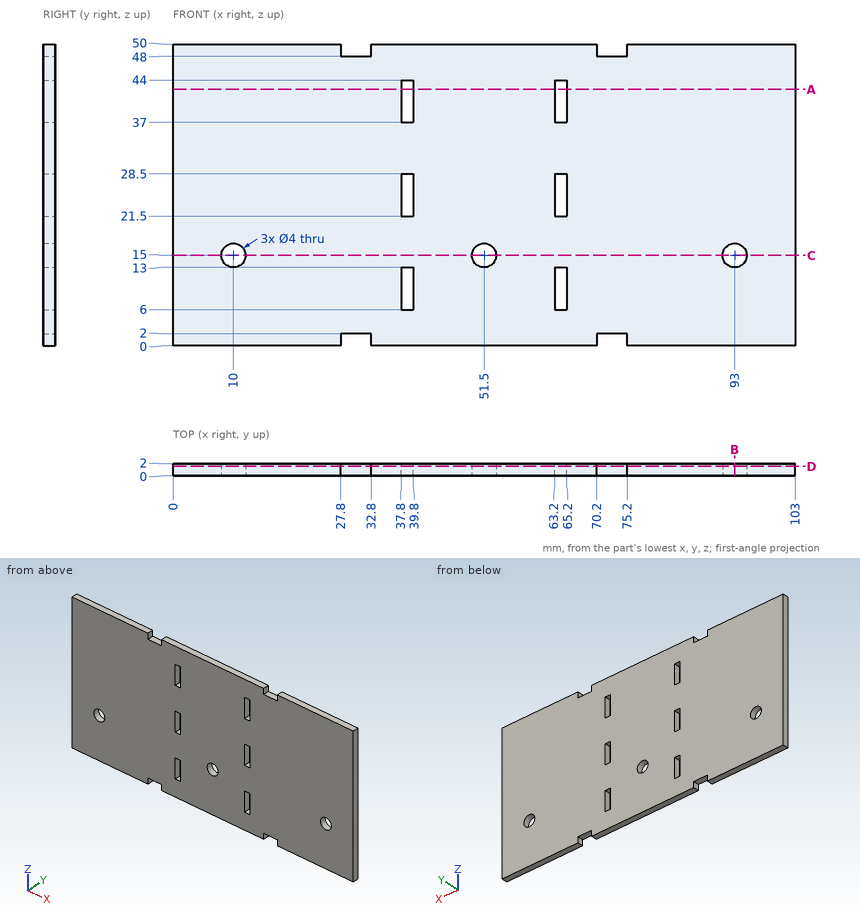
Geometry: see drawing. Coordinates: mm, zero at the bounding-box minimum. Give positions to 0.01 mm unless a question says otherwise; leave off trailing zeros. Loops run counter-clockwise (first coordinate to the right, second up) from the corner with the lowest first, then second, coordinate; pieces in that order, holes last. Notation, with made-up numbers: (62, 60.25) - (104, 60.25) arc R11 cw to (104, 67.25) - close; hole circle Ø3 at (51, 84). An arc over 180 degrees is marked (long way). Use CSV: the item, a comma, the result in double quotes.
1) Cut plane A-A (z = 42.5). Output: boundary loops of the cut face in (x, y), and give its area (3 significant figures).
Worked out:
outline,"(0, 0) - (37.8, 0) - (37.8, 2) - (0, 2) - close; (39.8, 0) - (63.2, 0) - (63.2, 2) - (39.8, 2) - close; (65.2, 0) - (103, 0) - (103, 2) - (65.2, 2) - close"
area,"198 mm^2"
2) Cut plane D-D (y = 1.6). Count the separate pieces of the cut face and the enclosed holes in it, and give its area (3 significant figures).
Worked out:
separate pieces,"1"
enclosed holes,"9"
area,"4,990 mm^2"
3) Cut plane C-C (z = 15). Output: boundary loops of the cut face in (x, y).
Worked out:
outline,"(0, 0) - (8, 0) - (8, 2) - (0, 2) - close; (12, 0) - (49.5, 0) - (49.5, 2) - (12, 2) - close; (53.5, 0) - (91, 0) - (91, 2) - (53.5, 2) - close; (95, 0) - (103, 0) - (103, 2) - (95, 2) - close"
4) Pin query (flat end, axial travel): P1, Ø1, axis at y = 1, z = 10.5, coming from the -X side; P2, Ø0.6, axis at x = 71.5, y = 1, coming from the +Z side. Return the tip coordinate at first contact, or that it passes through.
Worked out:
P1,"stops at x = 0"
P2,"stops at z = 48"
5) Cut plane B-B (x = 93). Output: boundary loops of the cut face in (y, z).
Worked out:
outline,"(0, 0) - (2, 0) - (2, 13) - (0, 13) - close; (0, 17) - (2, 17) - (2, 50) - (0, 50) - close"
6) Line query: line 1 (X direction, y = 0.15, z = 6.5); line 2 (X direction, y = 0.55, z = 15); line 3 (Z direction, x = 63.5, y = 1.5). Output: solid intervals per line, ascending.
Worked out:
line 1,"x = 0 to 37.8, 39.8 to 63.2, 65.2 to 103"
line 2,"x = 0 to 8, 12 to 49.5, 53.5 to 91, 95 to 103"
line 3,"z = 0 to 6, 13 to 21.5, 28.5 to 37, 44 to 50"
